Build history of the part. All positions in model axes, mm. Give positions to 0.01 mm unless a question says otherwise; leave off trailing zeros. Loops run counter-clockwise (first coordinate to the right, second up) from the corner with the lowest first, then second, coordinate; pieces in that order, holes last. Notation, with made-up numbers: (73.5, 61) -> (91.5, 61) arc R8 cw to (91.5, 67) -> close; hole circle Ø3 at (13.25, -19). An arc over 180 degrees is marked (long way). Answer as a JSON object with one key per item and string values. Group by question number.
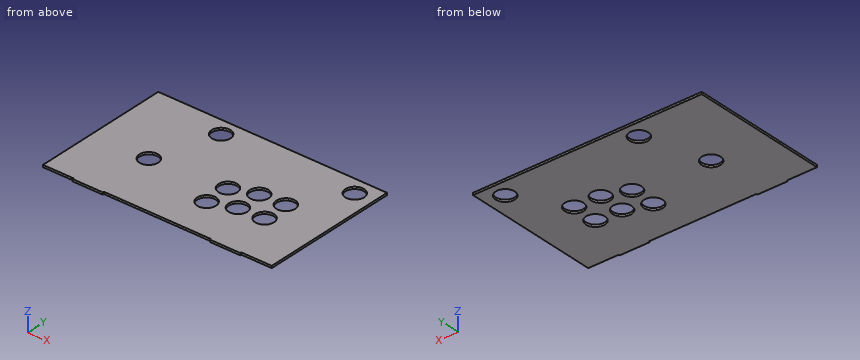
from build123d import *

# Parameters (mm, degrees)
F0_W     = 376
F0_H     = 227
F1_DEPTH = 3.5
F2_R     = 15.5
F3_DEPTH = 25
F5_W     = 50
F5_H     = 2
F6_DEPTH = 3.5


with BuildPart() as f1:
    # F0 (on Top) → F1 (new body)
    with BuildSketch(Plane.XY):
        with Locations((188, 113.5)):
            Rectangle(F0_W, F0_H)
    extrude(amount=F1_DEPTH)

    # F2 (on face) → F3 (cut)
    with BuildSketch(Plane.XY.offset(3.5)):
        with Locations((92.828363, 97.227663)):
            Circle(F2_R)
        with Locations((125.700176, 200.216234)):
            Circle(F2_R)
        with Locations((214.700887, 107.041298)):
            Circle(F2_R)
        with Locations((214.700887, 65.041298)):
            Circle(F2_R)
        with Locations((254.215892, 79.273809)):
            Circle(F2_R)
        with Locations((254.215892, 121.273809)):
            Circle(F2_R)
        with Locations((296.158493, 123.468865)):
            Circle(F2_R)
        with Locations((296.158493, 81.468865)):
            Circle(F2_R)
        with Locations((345.382124, 200.216234)):
            Circle(F2_R)
    extrude(amount=-F3_DEPTH, mode=Mode.SUBTRACT)

    # F5 (on face) → F6 (join)
    with BuildSketch(Plane.XY.offset(3.5)):
        with Locations((75, -1)):
            Rectangle(F5_W, F5_H)
        with Locations((301, -1)):
            Rectangle(F5_W, F5_H)
    extrude(amount=-F6_DEPTH)


solid = f1.part
(1) Saw through at B-B on z = 1.5. Give the number of separate pieces and of enclosed holes in the cut face, plus the area to 3 significant figures.
(2) Pin check, flat tips, straight feed: pin 1 (1.6 mm diameter, centred on y = -1, z = 2, fed in from -X); pin 2 (1.8 mm diameter, centred on x = 33, z = 1.5, fed in from -Y); pin 3 (1.6 mm diameter, centred on y = -1.5, z = 1.5, fed in from +X). Stop position of each tip, or through.
(3) Saw through at C-C on x = 219.5. List the corners of the cut face in (y, z).
(4) Saw through at A-A on y = 85.5. List the corners of the cut face in (x, z).
(5) Saw through at D-D on y = 194. List the corners of the cut face in (x, z).
(6) Probe line 1 along X through (y, z) = (199.5, 1.65); line 2 along Y through (x, z) = (288, 1.3); line 3 along Y through (x, z) = (261, 0.85). List the from-to ranges inside material, lowest first. Write a range as [from, to].
Calculated:
{
 "1": {"separate pieces": "1", "enclosed holes": "9", "area": "78,800 mm^2"},
 "2": {"pin 1": "stops at x = 50", "pin 2": "stops at y = 0", "pin 3": "stops at x = 326"},
 "3": {"outline": "(0, 0) -> (50.3, 0) -> (50.3, 3.5) -> (0, 3.5) -> close; (79.78, 0) -> (92.3, 0) -> (92.3, 3.5) -> (79.78, 3.5) -> close; (121.78, 0) -> (227, 0) -> (227, 3.5) -> (121.78, 3.5) -> close"},
 "4": {"outline": "(0, 0) -> (82.69, 0) -> (82.69, 3.5) -> (0, 3.5) -> close; (102.96, 0) -> (240.02, 0) -> (240.02, 3.5) -> (102.96, 3.5) -> close; (268.41, 0) -> (281.19, 0) -> (281.19, 3.5) -> (268.41, 3.5) -> close; (311.13, 0) -> (376, 0) -> (376, 3.5) -> (311.13, 3.5) -> close"},
 "5": {"outline": "(0, 0) -> (111.5, 0) -> (111.5, 3.5) -> (0, 3.5) -> close; (139.9, 0) -> (331.18, 0) -> (331.18, 3.5) -> (139.9, 3.5) -> close; (359.58, 0) -> (376, 0) -> (376, 3.5) -> (359.58, 3.5) -> close"},
 "6": {"line 1": "x = [0, 110.22], [141.18, 329.9], [360.87, 376]", "line 2": "y = [-2, 68.29], [94.65, 110.29], [136.65, 227]", "line 3": "y = [0, 65.34], [93.21, 107.34], [135.21, 227]"}
}
